from build123d import *

# Parameters (mm, degrees)
F1_DEPTH = 128
F3_DEPTH = 3.5
F4_R     = 2
F5_DEPTH = 6.051


with BuildPart() as f1:
    # F0 (on Front) → F1 (new body)
    with BuildSketch(Plane.XZ):
        Polygon((24.829483, 0), (44.829483, 0), (44.829483, 6.05), (26.579483, 6.05), (26.579483, 4.3), (24.829483, 4.3), align=None)
    extrude(amount=F1_DEPTH)

    # F2 (on face) → F3 (cut)
    with BuildSketch(Plane(origin=(0, 0, 0), x_dir=(1, 0, 0), z_dir=(0, 0, -1))):
        with BuildLine():
            ThreePointArc((32.329483, 117), (32.91527, 115.585786), (34.329483, 115))
            Line((34.329483, 115), (37.329483, 115))
            ThreePointArc((37.329483, 115), (38.743697, 115.585786), (39.329483, 117))
            Line((39.329483, 117), (39.329483, 121))
            ThreePointArc((39.329483, 121), (38.743697, 122.414214), (37.329483, 123))
            Line((37.329483, 123), (34.329483, 123))
            ThreePointArc((34.329483, 123), (32.91527, 122.414214), (32.329483, 121))
            Line((32.329483, 121), (32.329483, 117))
        make_face()
        with BuildLine():
            ThreePointArc((32.329483, 82), (32.91527, 80.585786), (34.329483, 80))
            Line((34.329483, 80), (37.329483, 80))
            ThreePointArc((37.329483, 80), (38.743697, 80.585786), (39.329483, 82))
            Line((39.329483, 82), (39.329483, 86))
            ThreePointArc((39.329483, 86), (38.743697, 87.414214), (37.329483, 88))
            Line((37.329483, 88), (34.329483, 88))
            ThreePointArc((34.329483, 88), (32.91527, 87.414214), (32.329483, 86))
            Line((32.329483, 86), (32.329483, 82))
        make_face()
        with BuildLine():
            ThreePointArc((37.329483, 40), (38.743697, 40.585786), (39.329483, 42))
            Line((39.329483, 42), (39.329483, 46))
            ThreePointArc((39.329483, 46), (38.743697, 47.414214), (37.329483, 48))
            Line((37.329483, 48), (34.329483, 48))
            ThreePointArc((34.329483, 48), (32.91527, 47.414214), (32.329483, 46))
            Line((32.329483, 46), (32.329483, 42))
            ThreePointArc((32.329483, 42), (32.91527, 40.585786), (34.329483, 40))
            Line((34.329483, 40), (37.329483, 40))
        make_face()
        with BuildLine():
            ThreePointArc((37.329483, 5), (38.743697, 5.585786), (39.329483, 7))
            Line((39.329483, 7), (39.329483, 11))
            ThreePointArc((39.329483, 11), (38.743697, 12.414214), (37.329483, 13))
            Line((37.329483, 13), (34.329483, 13))
            ThreePointArc((34.329483, 13), (32.91527, 12.414214), (32.329483, 11))
            Line((32.329483, 11), (32.329483, 7))
            ThreePointArc((32.329483, 7), (32.91527, 5.585786), (34.329483, 5))
            Line((34.329483, 5), (37.329483, 5))
        make_face()
    extrude(amount=-F3_DEPTH, mode=Mode.SUBTRACT)

    # F4 (on face) → F5 (cut, through all)
    with BuildSketch(Plane(origin=(0, 0, 0), x_dir=(1, 0, 0), z_dir=(0, 0, -1))):
        with Locations((35.829483, 119)):
            Circle(F4_R)
        with Locations((35.829483, 84)):
            Circle(F4_R)
        with Locations((35.829483, 44)):
            Circle(F4_R)
        with Locations((35.829483, 9)):
            Circle(F4_R)
    extrude(amount=-F5_DEPTH, mode=Mode.SUBTRACT)


solid = f1.part
Could you check a few things on this model? Use its own coordinates, in mm. A direction names the side the tool comes from. Give positions to 0.01 mm unless a question says otherwise; leave off trailing zeros. Order: outer loops, then holes, each group sorted by start corner. A loop starts at its lowest first (then second) coordinate and runs counter-clockwise, first axis right, second up.
Item 1: I'm going to push flat-ended pins straight in: pin 1 (2.5 mm diameter, centred on x = 35.5, z = 1.5, fed in from +Y); pin 2 (1.4 mm diameter, centred on x = 25.5, y = -70, fed in from +Z); pin 3 (3.5 mm diameter, centred on x = 36.5, y = -45, fed in from -Z). Where does each tip first touch, or does it pass through?
Item 2: For faces 5 (the face through (34.4, -10.4, 4.8)), 6 (the face through (32.9, -87.4, 1.7)), which set-ups out of +Z, -Z, +X, -X, +Y, -Y let a thin tool reach every point of the face, with its end or its side?
Item 3: If we mould it in two halves opening along X, with no side actions, what happens to faces 1 (the face through (35, -128, 3)), 2 (the face through (35.396, -42.048, 4.757)), 3 (the face through (44.829, -63, 3)), 4 (the face through (32.9, -115.6, 1.7))? For each: pulls with the +X half, pulls with the -X half, needs draft (parallel to the pull), parting line crosses it, or undercut.
Item 4: If we section it at B-B, the plane y = -52.5: Write out the boundary of the cut face in (x, z), plus the area to 3 significant figures.
Item 5: I need wall thicknesses on line 1 (Y direction, x = 34.75, z = 0.5); line 2 (X direction, y = -9, z = 5.45); line 3 (X direction, y = -10, z = 0.5). Which ranges of each line are inside material? Lowest first, please.
Item 6: If we section it at A-A, the plane y = -84: Write out the boundary of the cut face in (x, z), plus the area to 3 significant figures.
Item 7: If we section it at C-C, the plane z = 2: Count the separate pieces of the cut face and the enclosed holes in it, plus the area to 3 significant figures.
Values:
1. pin 1: stops at y = 0
1. pin 2: stops at z = 4.3
1. pin 3: stops at z = 3.5
2. face 5: +Z, -Z
2. face 6: -Z
3. face 1: needs draft
3. face 2: undercut
3. face 3: pulls with the +X half
3. face 4: undercut
4. outline: (24.83, 0) - (44.83, 0) - (44.83, 6.05) - (26.58, 6.05) - (26.58, 4.3) - (24.83, 4.3) - close
4. area: 118 mm2
5. line 1: y = -128 to -123, -115 to -88, -80 to -48, -40 to -13, -5 to 0
5. line 2: x = 26.58 to 33.83, 37.83 to 44.83
5. line 3: x = 24.83 to 32.33, 39.33 to 44.83
6. outline: (24.83, 0) - (32.33, 0) - (32.33, 3.5) - (33.83, 3.5) - (33.83, 6.05) - (26.58, 6.05) - (26.58, 4.3) - (24.83, 4.3) - close; (37.83, 3.5) - (39.33, 3.5) - (39.33, 0) - (44.83, 0) - (44.83, 6.05) - (37.83, 6.05) - close
6. area: 83.2 mm2
7. separate pieces: 1
7. enclosed holes: 4
7. area: 2,350 mm2
